The listing builds one solid part. Answer for the finished solid, in the listing's coordinates (mm). Round coordinates to 2 decimals unless told otherwise and drop trailing zeros. Put each result on its own line as item: value. Start each with the question number.
```python
from build123d import *

# Parameters (mm, degrees)
BOSS_EXTRUDE1_REACH = 28.188
SKETCH6_W           = 1.95
SKETCH6_H           = 0.55


# Read off the part's stored shape, not the designer's step: Revolve1
with BuildPart() as part:
    # Revolve1 outline → Revolve1 (revolve)
    with BuildSketch(Plane.XY):
        with BuildLine():
            Line((0, -3.048000121), (0, -6.747666043))
            ThreePointArc((0, -6.747666043), (2.031291213, -6.02834824), (3.157219843, -4.191000475))
            Line((3.157219843, -4.191000475), (3.175005592, -5.209936836))
            Line((3.175005592, -5.209936836), (3.175005592, -3.048000121))
            Line((3.175005592, -3.048000121), (0, -3.048000121))
        make_face()
        with BuildLine():
            ThreePointArc((3.047999762, -2.63e-07), (2.155261335, -2.155261626), (0, -3.048000121))
            Line((0, -3.048000121), (3.175005592, -3.048000121))
            Line((3.175005592, -3.048000121), (3.175005592, -2.63e-07))
            Line((3.175005592, -2.63e-07), (3.047999762, -2.63e-07))
        make_face()
        with BuildLine():
            Line((3.175005592, -3.048000121), (3.175005592, -5.209936836))
            Line((3.175005592, -5.209936836), (3.201846755, -6.747666043))
            Line((3.201846755, -6.747666043), (7.27518656, -6.747666043))
            add(Edge.make_bspline(
                [(7.27518656, -6.747666043), (7.21368894, -6.606752773), (6.964928048, -6.043911737), (6.546096871, -5.144737962), (6.026061135, -4.11883899), (5.658022957, -3.448984329), (5.463723236, -3.113412693), (5.425444316, -3.048000121)],
                knots=[0.445044946, 0.445044946, 0.445044946, 0.445044946, 0.477293423, 0.574115344, 0.653072781, 0.718507442, 0.734404118, 0.734404118, 0.734404118, 0.734404118], degree=3))
            Line((5.425444316, -3.048000121), (3.175005592, -3.048000121))
        make_face()
        with BuildLine():
            Line((3.175005592, -5.539e-06), (3.175005592, -3.048000121))
            Line((3.175005592, -3.048000121), (5.425444316, -3.048000121))
            add(Edge.make_bspline(
                [(5.425444316, -3.048000121), (5.331276728, -2.887082722), (5.120346092, -2.535848114), (4.796092557, -2.028683173), (4.466086303, -1.548435358), (4.165682257, -1.140937859), (3.890472725, -0.792449825), (3.569506506, -0.412648033), (3.330841371, -0.155867529), (3.175005592, -5.539e-06)],
                knots=[0.734404118, 0.734404118, 0.734404118, 0.734404118, 0.773510539, 0.820333182, 0.86064682, 0.895714403, 0.926505158, 0.95377342, 1, 1, 1, 1], degree=3))
        make_face()
        with BuildLine():
            Line((7.27518656, -6.747666043), (3.201846755, -6.747666043))
            Line((3.201846755, -6.747666043), (3.30574513, -12.7))
            Line((3.30574513, -12.7), (9.524999537, -12.7))
            add(Edge.make_bspline(
                [(9.524999537, -12.7), (8.986589512, -11.088985259), (8.268131113, -9.090761172), (7.444322602, -7.135217838), (7.27518656, -6.747666043)],
                knots=[0, 0, 0, 0, 0.356352413, 0.445044946, 0.445044946, 0.445044946, 0.445044946], degree=3))
        make_face()
    revolve(axis=Axis((0, 0, 0), (0, 1, 0)))

    # Sketch6 → Boss-Extrude1 (add, up to next)
    with BuildSketch(Plane(origin=(11.3025, 0, 0), x_dir=(0, 0, -1), z_dir=(1, 0, 0)), mode=Mode.PRIVATE) as boss_extrude1_sk1:
        with Locations((0, -12.425)):
            Rectangle(SKETCH6_W, SKETCH6_H)
    boss_extrude1_tool1 = extrude(boss_extrude1_sk1.sketch, amount=-BOSS_EXTRUDE1_REACH, mode=Mode.PRIVATE) - part.part
    boss_extrude1 = boss_extrude1_tool1.solids().sort_by_distance((11.3025, -12.425, 0))[0]
    add(boss_extrude1)

    # Mirror1: Boss-Extrude1 across plane
    add(boss_extrude1.mirror(Plane(origin=(0, 0, 0), x_dir=(0, 0, 1), z_dir=(1, 0, 0))))


solid = part.part
```
Item 1: Flat-ended cylindrical pins translate along their axes: pin 1 (1.5 mm diameter, centred on y = -1.5, z = -0.5, fed in from -X); pin 2 (5 mm diameter, centred on x = 7.5, z = -2, fed in from +Y); pin 3 (1 mm diameter, centred on x = -1.5, z = 1.5, fed in from -Y). Find the tip coordinate at first contact, or state that the pin passes through.
Item 2: Consider line 1 along X through (y, z) = (-7.75, -1.75); line 2 along X through (y, z) = (-8.25, 4.75); line 3 along Y through (x, z) = (6.25, -1.5). Determine where each line is inside the solid, lowest interval first. Write a range as [from, to].
Item 3: Section A-A (y = -6.25) is taken. Count the separate pieces of the cut face and the enclosed holes in it, and give its area (3 significant figures).
Output values:
1. pin 1: stops at x = -4.92
1. pin 2: stops at y = -2.77
1. pin 3: stops at y = -6.31
2. line 1: x = [-7.5, -2.7], [2.7, 7.5]
2. line 2: x = [-6.32, 6.32]
2. line 3: y = [-12.7, -4.92]
3. separate pieces: 2
3. enclosed holes: 1
3. area: 134 mm^2
